```python
from build123d import *

# Parameters (mm, degrees)
SKETCH_1_R          = 36.5
SKETCH_1_R_2        = 32.6
EXTRUDE_1_DEPTH     = 3.5
EXTRUDE_START       = 3
SKETCH_2_R          = 36.5
SKETCH_2_R_2        = 29.5
EXTRUDE_2_DEPTH     = 3
SKETCH_3_R          = 1.25
CUT_EXTRUDE_1_DEPTH = 20
CUT_EXTRUDE_2_DEPTH = 3


with BuildPart() as part:
    # 草图1 → 凸台-拉伸1 (new, symmetric)
    with BuildSketch(Plane.XY):
        Circle(SKETCH_1_R)
        Circle(SKETCH_1_R_2, mode=Mode.SUBTRACT)
    extrude(amount=EXTRUDE_1_DEPTH, both=True)

    # 草图2 → 凸台-拉伸2 (add)
    with BuildSketch(Plane.XY.offset(3.5).offset(EXTRUDE_START)):
        Circle(SKETCH_2_R)
        Circle(SKETCH_2_R_2, mode=Mode.SUBTRACT)
    extrude(amount=-EXTRUDE_2_DEPTH)

    # 草图3 → 切除-拉伸1 (cut)
    with BuildSketch(Plane(origin=(0, 0, -3.5), x_dir=(-1, 0, 0), z_dir=(0, 0, -1))):
        with Locations((0, 34)):
            Circle(SKETCH_3_R)
        with Locations((29.444863729, 17)):
            Circle(SKETCH_3_R)
        with Locations((29.444863729, -17)):
            Circle(SKETCH_3_R)
        with Locations((0, -34)):
            Circle(SKETCH_3_R)
        with Locations((-29.444863729, -17)):
            Circle(SKETCH_3_R)
        with Locations((-29.444863729, 17)):
            Circle(SKETCH_3_R)
    extrude(amount=-CUT_EXTRUDE_1_DEPTH, mode=Mode.SUBTRACT)

    # 草图4 → 切除-拉伸2 (cut)
    with BuildSketch(Plane.XY.offset(6.5)):
        Polygon((19.356134005, 221.241624062), (3.18118461, 36.36110648), (0, 0), (29.899049617, 20.935539927), (181.922799809, 127.383715799), (367.509530933, 448.829363315), (204.942865129, 542.687271578), align=None)
    extrude(amount=-CUT_EXTRUDE_2_DEPTH, mode=Mode.SUBTRACT)


solid = part.part
```
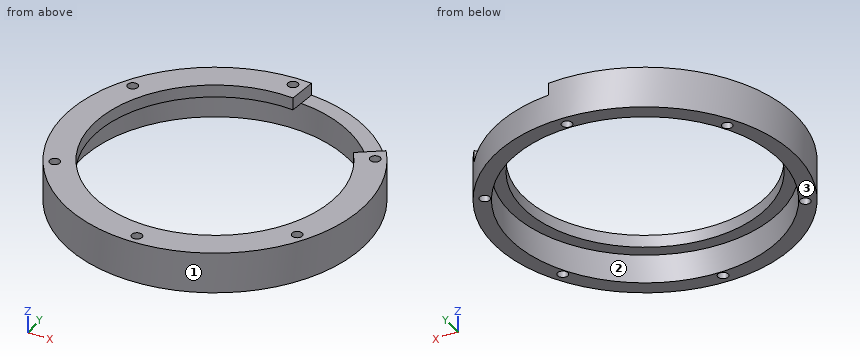
For this review, take the finished solid that the model builds, in its own axes (mm). Face numbers are marked on the shaded views. Coordinates: 2 decimals unless noted, no trailing zeros. Write each loop counter-clockwise with the first axis right and the second up, starting at its lowest first coordinate (ties: lowest second). Pieces come first, ordered by that corner, then holes.
(1) Add section C-C on z = -2.5. Give the boundary of the cut face in (x, y).
(2) For pin 1 Ø1.5 at (x, z) = (9.5, 1.5) entering from -Y; pin 2 Ø5 at (y, z) = (6, -1) entering from -X; pin 3 Ø2 at (x, y) = (-29.44, 17) entering from -Z; pin 4 Ø1 at (y, z) = (-10.5, 2) entering from +X, all flat-tipped, find the tip position at first contact; note any pin that passes through.
(3) The part is to be moulded in two halves that separate along X. For the marked faces 1, 2 and 3, say which applies: +X half, -X half, draft (parallel to the pull), parting line (faces both ways), or undercut.
(4) Add section A-A on x = 0. Give the boundary of the cut face in (y, z), then the cut area to 3 significant figures.
(5) Add section B-B on y = 0. Give the boundary of the cut face in (x, z).
(6) Add section D-D on x = 12. Give the boundary of the cut face in (y, z), then the cut area to 3 significant figures.
(7) Wall thickness on probe 1 along Y at (x, z) = (0, -1); probe 2 along X at (y, z) = (0, 1.5); probe 3 along X at (y, z) = (0, 4.6): over which ranges is each line inside the solid? List them lowest first.
Answer sheet:
1. outline: circle Ø73 at (0, 0); hole circle Ø65.2 at (0, 0); hole circle Ø2.5 at (-29.44, -17); hole circle Ø2.5 at (-29.44, 17); hole circle Ø2.5 at (0, -34); hole circle Ø2.5 at (0, 34); hole circle Ø2.5 at (29.44, -17); hole circle Ø2.5 at (29.44, 17)
2. pin 1: stops at y = -35.44
2. pin 2: stops at x = -36.33
2. pin 3: passes through
2. pin 4: stops at x = 35.1
3. face 1: parting line
3. face 2: undercut
3. face 3: draft
4. outline: (-36.5, -3.5) - (-35.25, -3.5) - (-35.25, 6.5) - (-36.5, 6.5) - close; (-32.75, -3.5) - (-32.6, -3.5) - (-32.6, 3.5) - (-29.5, 3.5) - (-29.5, 6.5) - (-32.75, 6.5) - close; (29.5, 3.5) - (32.6, 3.5) - (32.6, -3.5) - (32.75, -3.5) - (32.75, 6.5) - (29.5, 6.5) - close; (35.25, -3.5) - (36.5, -3.5) - (36.5, 6.5) - (35.25, 6.5) - close
4. area: 46.6 mm2
5. outline: (-36.5, -3.5) - (-32.6, -3.5) - (-32.6, 3.5) - (-29.5, 3.5) - (-29.5, 6.5) - (-36.5, 6.5) - close; (29.5, 3.5) - (32.6, 3.5) - (32.6, -3.5) - (36.5, -3.5) - (36.5, 6.5) - (29.5, 6.5) - close
6. outline: (-34.47, -3.5) - (-30.31, -3.5) - (-30.31, 3.5) - (-26.95, 3.5) - (-26.95, 6.5) - (-34.47, 6.5) - close; (30.31, -3.5) - (34.47, -3.5) - (34.47, 3.5) - (30.31, 3.5) - close
6. area: 80.8 mm2
7. probe 1: y = -36.5 to -35.25, -32.75 to -32.6, 32.6 to 32.75, 35.25 to 36.5
7. probe 2: x = -36.5 to -32.6, 32.6 to 36.5
7. probe 3: x = -36.5 to -29.5, 29.5 to 36.5
